The model under review builds one solid part; all positions refer to its coordinate system, in mm. A direction names the side the tool comes from. Give positions to 0.01 mm unless a question says otherwise; leave off trailing zeros. Loops run counter-clockwise (first coordinate to the right, second up) from the corner with the lowest first, then second, coordinate; pieces in that order, holes last. Notation, with made-up numbers: (62.5, 25) - (96.5, 25) arc R23 cw to (96.5, 40) - close; hole circle Ø8 at (77, 16.5). An arc over 180 degrees is marked (long way). Return JSON: item names as keys, results as strings. Group by question number.
```python
from build123d import *

# Parameters (mm, degrees)
F0_R     = 8.5
F1_DEPTH = 4
F2_R     = 5
F3_DEPTH = 100
F6_R     = 1.5
F7_DEPTH = 123


with BuildPart() as f1:
    # F0 (on Top) → F1 (new body)
    with BuildSketch(Plane.XY):
        Circle(F0_R)
    extrude(amount=F1_DEPTH)

    # F2 (on Top) → F3 (join)
    with BuildSketch(Plane.XY):
        Circle(F2_R)
    extrude(amount=F3_DEPTH)

    # F4 (on Right) → F5 (revolve)
    with BuildSketch(Plane.YZ):
        Polygon((3, 105), (0, 105), (0, 100), (4, 100), align=None)
    revolve(axis=Axis((0, 0, 102.5), (0, 0, -1)))

    # F6 (on face) → F7 (cut)
    with BuildSketch(Plane.XY.offset(105)):
        Circle(F6_R)
    extrude(amount=-F7_DEPTH, mode=Mode.SUBTRACT)


solid = f1.part
```
1) We need section A-A, the plane x = 0. Write out the cut boundary in (y, z), plus the area to 3 significant figures.
2) We need section C-C, the plane x = -7.5. Write out the cut boundary in (y, z), plus the area to 3 significant figures.
3) We need section B-B, the plane z = 59. Write out the cut boundary in (x, y), plus the area to 3 significant figures.
4) To check wall thickness, follow line 1 (Y direction, x = 0, z = 49); line 2 (X direction, y = 3, z = 61); line 3 (Z direction, x = 3.5, y = 6.5). State the ranges of each line that lie inside material, in increasing order.
5) We need section D-D, the plane x = 6.75. Write out the cut boundary in (y, z).
6) Draft analysis for pull direction X (two halves, no side actions). For faces 3 (the face through (-1.5, 0.07, 53.24)), 4 (the face through (-1.3, 1.3, 105)), 5 (the face through (-1.08, -4.88, 51.33)), state which applies: +X half, -X half, draft (parallel to the pull), parting line (faces both ways), or undercut.
7) Tool access review of faces 1 (the face through (4, -4, 4)), 2 (the face through (2, 0, 0)): name each direction out of +Z, -Z, +X, -X, +Y, -Y from which nothing blocks a thin tool from reaching the whole face with its end or side.
8) For pin 1 Ø4 at (y, z) = (4.5, 72) entering from -X; pin 2 Ø4 at (x, y) = (-4, -1.5) entering from -Z; pin 3 Ø3 at (x, y) = (-6, 6) entering from +Z; pin 4 Ø6 at (y, z) = (-0.5, 27) entering from +X, all flat-tipped, find the tip position at first contact; note any pin that passes through.
Findings:
{
 "1": {"outline": "(-8.5, 0) - (-1.5, 0) - (-1.5, 105) - (-3, 105) - (-4, 100) - (-5, 100) - (-5, 4) - (-8.5, 4) - close; (1.5, 0) - (8.5, 0) - (8.5, 4) - (5, 4) - (5, 100) - (4, 100) - (3, 105) - (1.5, 105) - close", "area": "748 mm^2"},
 "2": {"outline": "(-4, 0) - (4, 0) - (4, 4) - (-4, 4) - close", "area": "32.0 mm^2"},
 "3": {"outline": "circle Ø10 at (0, 0); hole circle Ø3 at (0, 0)", "area": "71.5 mm^2"},
 "4": {"line 1": "y = -5 to -1.5, 1.5 to 5", "line 2": "x = -4 to 4", "line 3": "z = 0 to 4"},
 "5": {"outline": "(-5.17, 0) - (5.17, 0) - (5.17, 4) - (-5.17, 4) - close"},
 "6": {"face 3": "undercut", "face 4": "draft", "face 5": "parting line"},
 "7": {"face 1": "+Z", "face 2": "-Z, +X, -X, +Y, -Y"},
 "8": {"pin 1": "stops at x = -4.33", "pin 2": "stops at z = 0", "pin 3": "stops at z = 4", "pin 4": "stops at x = 5"}
}
